Drawing for the job (mm, zero at the part's lowest x, y, z). A direction names the side the tool comes from. Give positions to 0.01 mm unless a question says otherwise; leave off trailing zeros. Order: outer loops, then holes, each group sorted by start corner. A loop starts at its lowest first (then second) coordinate and runs counter-clockwise, first axis right, second up. Notation, with made-up numbers: (-19.75, -36.75) -> (38.25, -36.75) arc R12 cw to (38.25, -30.75) -> close; hole circle Ø6 at (6, 68). An arc over 180 degrees is marked (long way). Use one line per item in the form item = value. Start each with the question number.
1) Cut at A-A, the plane y = 30. Give the cut face in (x, z), and give its area (3 significant figures).
2) Mould opens along Y. For the marked faces 1, 2 and 3 say: pulls with the +Y half, pulls with the -Y half, needs draft (parallel to the pull), parting line crosses it, or undercut.
3) Tool access for the marked faces 4, 5 and 6: list every direction of +Z, -Z, +X, -X, +Y, -Y with a clear straight run to the whole face (end or side of a thin tool).
4) Drop flat-ended pins along their axis: P1, Ø5, axis at x = 18.5, y = 53.5, coming from the +Z side; P2, Ø1, axis at x = 14, z = 12, coming from the -Y side; P3, Ø3, axis at y = 38.5, z = 45, coming from the -X side. Give the stop position or say it passes through.
5) Cut at B-B, the plane z = 57.5. Give the cut face in (x, y).
6) Cut at C-C, the plane x = 36. Give the cut face in (y, z).
7) Probe line 1 (Y direction, x = 30, z = 11); line 2 (X direction, y = 29, z = 48). List the from-to ranges inside material, lowest first.
8) Cut at D-D, the plane y = 5. Give the cut face in (x, z).
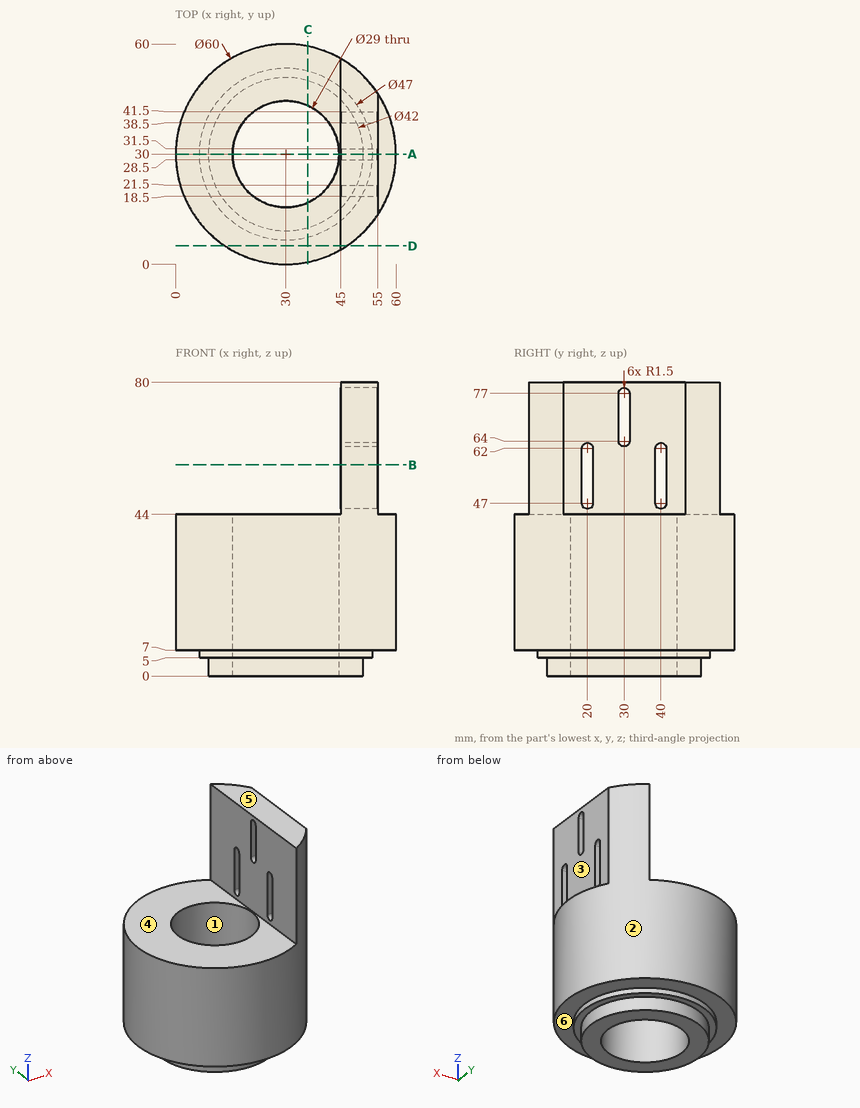
Result:
q1.outline = (0, 7) -> (6.5, 7) -> (6.5, 5) -> (9, 5) -> (9, 0) -> (15.5, 0) -> (15.5, 44) -> (0, 44) -> close; (44.5, 0) -> (51, 0) -> (51, 5) -> (53.5, 5) -> (53.5, 7) -> (60, 7) -> (60, 44) -> (55, 44) -> (55, 62.5) -> (45, 62.5) -> (45, 44) -> (44.5, 44) -> close; (45, 78.5) -> (55, 78.5) -> (55, 80) -> (45, 80) -> close
q1.area = 1,450 mm²
q2.face_1 = undercut
q2.face_2 = parting line crosses it
q2.face_3 = needs draft
q3.face_4 = +Z, -X, +Y, -Y
q3.face_5 = +Z, +X, -X, +Y, -Y
q3.face_6 = -Z
q4.P1 = 44
q4.P2 = 4.31
q4.P3 = 0.92
q5.outline = (45, 4.02) arc R30 ccw to (55, 13.42) -> (55, 18.5) -> (45, 18.5) -> close; (45, 21.5) -> (55, 21.5) -> (55, 38.5) -> (45, 38.5) -> close; (45, 41.5) -> (55, 41.5) -> (55, 46.58) arc R30 ccw to (45, 55.98) -> close
q6.outline = (0.61, 7) -> (7.28, 7) -> (7.28, 5) -> (9.88, 5) -> (9.88, 0) -> (16.8, 0) -> (16.8, 44) -> (0.61, 44) -> close; (43.2, 0) -> (50.12, 0) -> (50.12, 5) -> (52.72, 5) -> (52.72, 7) -> (59.39, 7) -> (59.39, 44) -> (43.2, 44) -> close
q7.line_1 = 0 to 15.5, 44.5 to 60
q7.line_2 = 45 to 55
q8.outline = (13.42, 7) -> (46.58, 7) -> (46.58, 80) -> (45, 80) -> (45, 44) -> (13.42, 44) -> close
